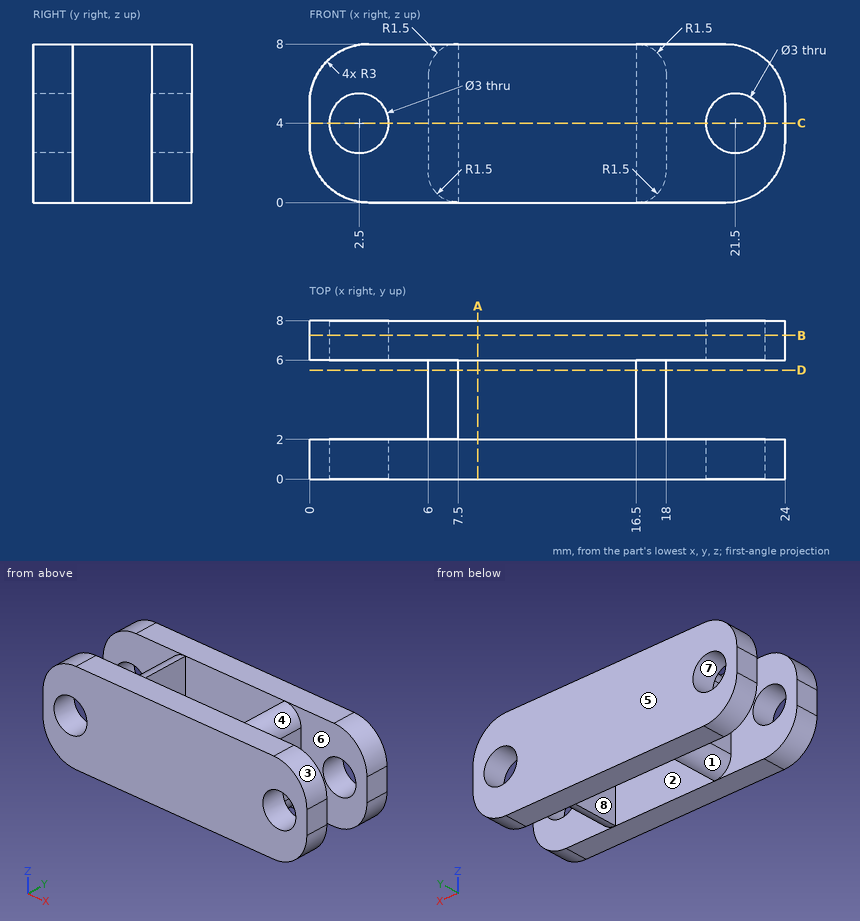
For this review, use the dimensioned drawing (mm, ordinates from the lowest corner) and the shaded views. A direction names the side the tool comes from. Round coordinates to 2 decimals unless told otherwise and drop trailing zeros. Order: outer loops, then holes, each group sorted by start corner. A loop starts at its lowest first (then second) coordinate and runs counter-clockwise, first axis right, second up. Notation, with made-up numbers: M 55,46 L 112,46 A20 cw 112,57 Z; hole C -38.75,30.25 d2. An arc over 180 degrees is marked long. Use a Markdown table: item, result. Add a question column.
Item 1: Insertion check: pin 1 (4 mm diameter, centred on x = 19.5, z = 5.5, fed in from -Y); pin 2 (1 mm diameter, centred on x = 13.5, y = 5, fed in from +Z); pin 3 (1.2 mm diameter, centred on y = 5, z = 5.5, fed in from +X); pin 4 (2 mm diameter, centred on y = 4, z = 2, fed in from -X). Each pin has a flat end and moves straight along its axis. Give the tip position at first contact, or say it passes through.
Item 2: Mouldability with a two-part tool opening along Y and no side actions: class the marked faces 5, 6, 7 and 8 as released by +Y, released by -Y, zero draft, split by the parting line, or undercut.
Item 3: Add section C-C, the plane z = 4. State how many separate pieces and enclosed holes the cut face has, then the cut area to 3 significant figures.
Item 4: Add section D-D, the plane y = 5.5. Give the boundary of the cut face in (x, z), then the cut area to 3 significant figures.
Item 5: Tool access review of the marked faces 1, 2, 3 and 4: name each direction out of +Z, -Z, +X, -X, +Y, -Y from which nothing blocks a thin tool from reaching the whole face with its end or side.
Item 6: Add section A-A, the plane x = 8.5. Give the boundary of the cut face in (y, z), then the cut area to 3 significant figures.
Item 7: To check wall thickness, follow line 1 along Y through (x, z) = (16, 3.25); line 2 along X through (y, z) = (0.5, 4.5); line 3 along Z through (x, y) = (2.5, 0.8). State the ranges of each line that lie inside material, in increasing order.
Item 8: Add section B-B, the plane y = 7.25. Give the boundary of the cut face in (x, z).
Geometry results:
| question | item | result |
|---|---|---|
| 1 | pin 1 | stops at y = 0 |
| 1 | pin 2 | passes through |
| 1 | pin 3 | stops at x = 18 |
| 1 | pin 4 | stops at x = 6 |
| 2 | face 5 | released by +Y |
| 2 | face 6 | undercut |
| 2 | face 7 | zero draft |
| 2 | face 8 | undercut |
| 3 | separate pieces | 5 |
| 3 | enclosed holes | 1 |
| 3 | area | 84.0 mm² |
| 4 | outline | M 6,1.5 A1.5 ccw 7.5,0 L 7.5,8 A1.5 ccw 6,6.5 Z; M 16.5,0 A1.5 ccw 18,1.5 L 18,6.5 A1.5 ccw 16.5,8 Z |
| 4 | area | 22.1 mm² |
| 5 | face 1 | -Z, -X |
| 5 | face 2 | +Z, -Z |
| 5 | face 3 | +Z, +X, +Y, -Y |
| 5 | face 4 | +Z, +X |
| 6 | outline | M 0,0 L 2,0 L 2,8 L 0,8 Z; M 6,0 L 8,0 L 8,8 L 6,8 Z |
| 6 | area | 32.0 mm² |
| 7 | line 1 | y = 0 to 2, 6 to 8 |
| 7 | line 2 | x = 0 to 1.09, 3.91 to 20.09, 22.91 to 24 |
| 7 | line 3 | z = 0.04 to 2.5, 5.5 to 7.96 |
| 8 | outline | M 0,3 A3 ccw 3,0 L 21,0 A3 ccw 24,3 L 24,5 A3 ccw 21,8 L 3,8 A3 ccw 0,5 Z; hole C 2.5,4 d3; hole C 21.5,4 d3 |
